Could you check a few things on this drawing? It's one solid part, dimensions in mm from its lowest x, y, z. A direction names the side the tool comes from. Coordinates: 2 decimals unless noted, no trailing zeros. Loops run counter-clockwise (first coordinate to the right, second up) from the corner with the lowest first, then second, coordinate; pieces in that order, holes last.
1) Imagine slicing it at D-D on z = 7.5. Please give me the cut outline in (x, y).
2) Imagine slicing it at C-C on x = 23. Please give me the cut outline in (y, z).
3) Thinking about a two-plate mould opening in Y: for the marked faces 3, 4, 5 and 6, which applies, released by +Y, released by -Y, zero draft, split by the parting line, or undercut?
4) Will these pins go through, and if not, where does the flat tip stop? P1, Ø10, axis at x = 7.5, y = 6, coming from the -Z side; P2, Ø2.5, axis at y = 11, z = 4, coming from the -X side; P3, Ø4, axis at x = 10, z = 5, coming from the +Y side.
5) Imagine slicing it at B-B on y = 4. Please give me the cut outline in (x, z), plus the area to 3 significant figures.
6) Imagine slicing it at A-A on z = 4. Please give me the cut outline in (x, y).
7) If I drill on line 1 along Y through (x, z) = (23.5, 4); line 2 along X through (y, z) = (16, 3.5); line 3 along Y through (x, z) = (24.5, 2.5), over which ranges is the centre line in solid material (lowest first)?
8) For the marked faces 1 and 2, which set-ups out of +Z, -Z, +X, -X, +Y, -Y let a thin tool reach every point of the face, with its end or its side?
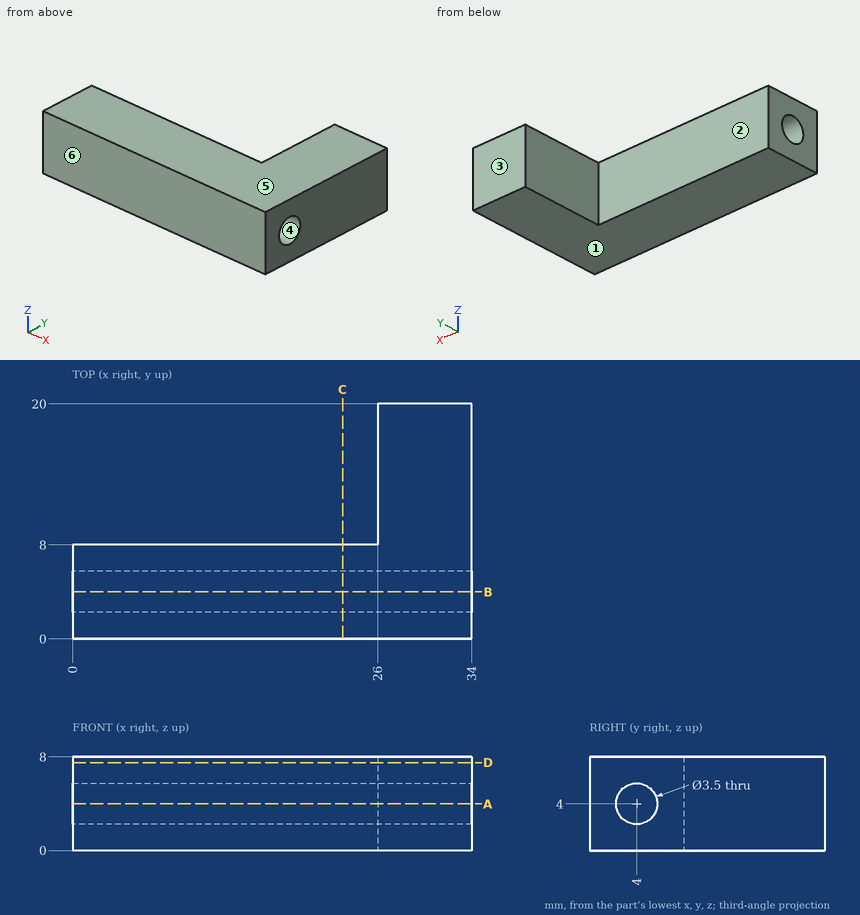
Filled in:
1. outline: (0, 0) - (34, 0) - (34, 20) - (26, 20) - (26, 8) - (0, 8) - close
2. outline: (0, 0) - (8, 0) - (8, 8) - (0, 8) - close; hole circle Ø3.5 at (4, 4)
3. face 3: released by +Y
3. face 4: undercut
3. face 5: zero draft
3. face 6: released by -Y
4. P1: stops at z = 0
4. P2: stops at x = 26
4. P3: stops at y = 8
5. outline: (0, 0) - (34, 0) - (34, 2.25) - (0, 2.25) - close; (0, 5.75) - (34, 5.75) - (34, 8) - (0, 8) - close
5. area: 153 mm2
6. outline: (0, 0) - (34, 0) - (34, 2.25) - (0, 2.25) - close; (0, 5.75) - (34, 5.75) - (34, 20) - (26, 20) - (26, 8) - (0, 8) - close
7. line 1: y = 0 to 2.25, 5.75 to 8
7. line 2: x = 26 to 34
7. line 3: y = 0 to 3.1, 4.9 to 8
8. face 1: -Z, +X, -X, +Y, -Y
8. face 2: +Z, -Z, -X, +Y
